Here's how the part is built. I have some questions about the finished solid (model axes, mm). Round coordinates to 2 decimals unless told otherwise and drop trailing zeros. Write each loop counter-clockwise with the first axis right and the second up, starting at its lowest first coordinate (ties: lowest second). Pieces come first, ordered by that corner, then holes. Notation, with made-up numbers: (-12, -34) - (-3, -34) arc R32 ccw to (-3, -6) - close; hole circle Ø3 at (53, 2). An arc over 180 degrees is marked (long way). Use one line per item in the form item = value. Start each with the question number.
1. If I drill on line 1 along Y through (x, z) = (-51, 0.7); line 2 along X through (y, z) = (-20, 0.6); line 3 along X through (y, z) = (-11, 1.45), over which ranges is the centre line in solid material (lowest first)?
2. I want a section at A-A, the plane y = 9. List the corners of the cut face in (x, z) for me, plus the area to 3 significant figures.
3. I want a section at C-C, the plane x = -97. List the corners of the cut face in (y, z) for me, plus the area to 3 significant figures.
4. I want a section at D-D, the plane z = 4.05. State how many separate pieces and enclosed holes the cut face has, plus the area to 3 significant figures.
5. I want a section at B-B, the plane x = -58. List the corners of the cut face in (y, z) for me, plus the area to 3 significant figures.
6. Will this pin go through, and if not, where does the flat tip stop? pin 1 (12 mm diameter, centred on x = -73.77, y = -20.19, fed in from -Z).
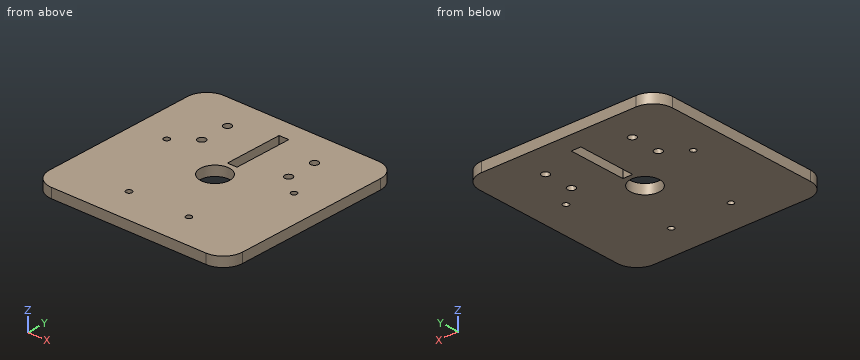
```python
from build123d import *

# Parameters (mm, degrees)
CROQUIS1_W              = 100
CROQUIS1_H              = 100
CROQUIS1_R              = 7.5
CROQUIS1_W_2            = 5
CROQUIS1_H_2            = 30
SALIENTE_EXTRUIR1_DEPTH = 5
REDONDEO1_R             = 10
CROQUIS3_R              = 1.5
CROQUIS3_R_2            = 1.500000006
CORTAR_EXTRUIR1_DEPTH   = 5
CORTAR_EXTRUIR2_REACH   = 144.377
CROQUIS4_R              = 2


with BuildPart() as part:
    # Croquis1 → Saliente-Extruir1 (new body)
    with BuildSketch(Plane.XY):
        with Locations((-73.773233416, -20.188160544)):
            Rectangle(CROQUIS1_W, CROQUIS1_H)
        with Locations((-73.773233416, -20.188160544)):
            Circle(CROQUIS1_R, mode=Mode.SUBTRACT)
        with Locations((-73.773233416, 4.811839456)):
            Rectangle(CROQUIS1_W_2, CROQUIS1_H_2, mode=Mode.SUBTRACT)
    extrude(amount=SALIENTE_EXTRUIR1_DEPTH)

    # Redondeo1
    redondeo1_edges = [part.edges().sort_by_distance(p)[0] for p in [
        (-23.773233416, 29.811839456, 2.5),
        (-23.773233416, -70.188160544, 2.5),
        (-123.773233416, -70.188160544, 2.5),
        (-123.773233416, 29.811839456, 2.5),
    ]]
    fillet(redondeo1_edges, radius=REDONDEO1_R)

    # Croquis3 → Cortar-Extruir1 (cut)
    with BuildSketch(Plane(origin=(0, 0, 0), x_dir=(-1, 0, 0), z_dir=(0, 0, -1))):
        with Locations((106.757827558, -11.251647632)):
            Circle(CROQUIS3_R)
        with Locations((40.788639233, -11.251647632)):
            Circle(CROQUIS3_R_2)
        with Locations((89.273233395, -52.688161005)):
            Circle(CROQUIS3_R)
        with Locations((58.273233395, -52.688161005)):
            Circle(CROQUIS3_R)
    extrude(amount=-CORTAR_EXTRUIR1_DEPTH, mode=Mode.SUBTRACT)

    # Croquis4 → Cortar-Extruir2 (cut, up to next)
    with BuildSketch(Plane.XY.offset(5), mode=Mode.PRIVATE) as cortar_extruir2_sk1:
        with Locations((-51.273233416, 12.311839456)):
            Circle(CROQUIS4_R)
    cortar_extruir2_tool1 = extrude(cortar_extruir2_sk1.sketch, amount=-CORTAR_EXTRUIR2_REACH, mode=Mode.PRIVATE) & part.part
    # Croquis4 → Cortar-Extruir2 (cut, up to next)
    with BuildSketch(Plane.XY.offset(5), mode=Mode.PRIVATE) as cortar_extruir2_sk2:
        with Locations(Location((-96.273233416, 12.311839456, 0), (0, 0, 180))):
            Circle(CROQUIS4_R)
    cortar_extruir2_tool2 = extrude(cortar_extruir2_sk2.sketch, amount=-CORTAR_EXTRUIR2_REACH, mode=Mode.PRIVATE) & part.part
    # Croquis4 → Cortar-Extruir2 (cut, up to next)
    with BuildSketch(Plane.XY.offset(5), mode=Mode.PRIVATE) as cortar_extruir2_sk3:
        with Locations((-96.273233416, -2.688160544)):
            Circle(CROQUIS4_R)
    cortar_extruir2_tool3 = extrude(cortar_extruir2_sk3.sketch, amount=-CORTAR_EXTRUIR2_REACH, mode=Mode.PRIVATE) & part.part
    # Croquis4 → Cortar-Extruir2 (cut, up to next)
    with BuildSketch(Plane.XY.offset(5), mode=Mode.PRIVATE) as cortar_extruir2_sk4:
        with Locations(Location((-51.273233416, -2.688160544, 0), (0, 0, 180))):
            Circle(CROQUIS4_R)
    cortar_extruir2_tool4 = extrude(cortar_extruir2_sk4.sketch, amount=-CORTAR_EXTRUIR2_REACH, mode=Mode.PRIVATE) & part.part
    add(cortar_extruir2_tool1.solids().sort_by_distance((-51.273233, 12.311839, 5))[0], mode=Mode.SUBTRACT)
    add(cortar_extruir2_tool2.solids().sort_by_distance((-96.273233, 12.311839, 5))[0], mode=Mode.SUBTRACT)
    add(cortar_extruir2_tool3.solids().sort_by_distance((-96.273233, -2.688161, 5))[0], mode=Mode.SUBTRACT)
    add(cortar_extruir2_tool4.solids().sort_by_distance((-51.273233, -2.688161, 5))[0], mode=Mode.SUBTRACT)


solid = part.part
```
Model answer:
q1.line_1 = -70.19 to -4.67, -0.71 to 10.33, 14.29 to 29.81
q1.line_2 = -123.77 to -81.27, -66.28 to -23.77
q1.line_3 = -123.77 to -108.24, -105.28 to -42.27, -39.31 to -23.77
q2.outline = (-123.77, 0) - (-76.27, 0) - (-76.27, 5) - (-123.77, 5) - close; (-71.27, 0) - (-23.77, 0) - (-23.77, 5) - (-71.27, 5) - close
q2.area = 475 mm2
q3.outline = (-70.19, 0) - (-4.55, 0) - (-4.55, 5) - (-70.19, 5) - close; (-0.82, 0) - (10.45, 0) - (10.45, 5) - (-0.82, 5) - close; (14.18, 0) - (29.81, 0) - (29.81, 5) - (14.18, 5) - close
q3.area = 463 mm2
q4.separate_pieces = 1
q4.enclosed_holes = 10
q4.area = 9,510 mm2
q5.outline = (-70.19, 0) - (-54.16, 0) - (-54.16, 5) - (-70.19, 5) - close; (-51.21, 0) - (29.81, 0) - (29.81, 5) - (-51.21, 5) - close
q5.area = 485 mm2
q6.pin_1 = through
